```python
from build123d import *

# Parameters (mm, degrees)
SKETCH_1_R          = 6
EXTRUDE_1_DEPTH     = 3
FILLET_1_R          = 2
SKETCH_2_R          = 1.515
CUT_EXTRUDE_1_DEPTH = 10
CUT_EXTRUDE_2_DEPTH = 10
FILLET_2_R          = 1.2


with BuildPart() as part:
    # 草图1 → 凸台-拉伸1 (new body)
    with BuildSketch(Plane.XY):
        with BuildLine():
            Line((-20, -45), (20, -45))
            Line((20, -45), (20, -39))
            Line((20, -39), (12.287533689, 2.294889071))
            ThreePointArc((12.287533689, 2.294889071), (0, 12.5), (-12.287533689, 2.294889071))
            Line((-12.287533689, 2.294889071), (-20, -39))
            Line((-20, -39), (-20, -45))
        make_face()
        Circle(SKETCH_1_R, mode=Mode.SUBTRACT)
    extrude(amount=EXTRUDE_1_DEPTH)

    # 圆角1
    fillet_1_edges = [part.edges().sort_by_distance(p)[0] for p in [
        (20, -39, 1.5),
        (20, -45, 1.5),
        (-20, -45, 1.5),
        (-20, -39, 1.5),
    ]]
    fillet(fillet_1_edges, radius=FILLET_1_R)

    # 草图2 → 切除-拉伸1 (cut)
    with BuildSketch(Plane.XY.offset(3)):
        with Locations((-5, -42)):
            Circle(SKETCH_2_R)
        with Locations((15, -42)):
            Circle(SKETCH_2_R)
    extrude(amount=-CUT_EXTRUDE_1_DEPTH, mode=Mode.SUBTRACT)

    # 草图3 → 切除-拉伸2 (cut)
    with BuildSketch(Plane.XY.offset(3)):
        with BuildLine():
            Line((-8.849829987, -6.53303216), (-14.913543956, -39))
            Line((-14.913543956, -39), (14.913543956, -39))
            Line((14.913543956, -39), (8.849829987, -6.53303216))
            ThreePointArc((8.849829987, -6.53303216), (0, -11), (-8.849829987, -6.53303216))
        make_face()
    extrude(amount=-CUT_EXTRUDE_2_DEPTH, mode=Mode.SUBTRACT)

    # 圆角2
    fillet_2_edges = [part.edges().sort_by_distance(p)[0] for p in [
        (-8.849829987, -6.53303216, 1.5),
        (8.849829987, -6.53303216, 1.5),
        (14.913543956, -39, 1.5),
        (-14.913543956, -39, 1.5),
    ]]
    fillet(fillet_2_edges, radius=FILLET_2_R)


solid = part.part
```
Input: part model. Units: mm. Frame: model coordinates. A direction names the side the tool comes from. Round coordinates to 2 decimals unless told otherwise and drop trailing zeros. Write each loop counter-clockwise with the first axis right and the second up, starting at its lowest first coordinate (ties: lowest second). Pieces come first, ordered by that corner, then holes. Notation, with made-up numbers: M 50,39.5 L 73,39.5 A13 ccw 73,46.5 Z; hole C 71,-38 d7. An arc over 180 degrees is marked long. Write each question's results on one line, items separated by ' | '.
Q1. Access query for faces 1 (the face through (0, -11, 2)), 2 (the face through (20, -41, 1)). Directions: +Z, -Z, +X, -X, +Y, -Y. A direction counts if a zero-diameter tool reaches every point of the face in a straight line with its end or side. Return the directions, or none.
Results:
face 1: +Z, -Z | face 2: +Z, -Z, +X, +Y, -Y
Q2. Draft query along X for faces 3 (the face through (-19.4, -44.43, 1.52)), 4 (the face through (0, -39, 2)), 5 (the face through (0, -9, 0)). Return one class per face: released by +X, released by -X, zero draft, split by the parting line, or undercut.
Results:
face 3: released by -X | face 4: undercut | face 5: zero draft
Q3. Line query: line 1 along Y through (x, z) = (0, 1.7); line 2 along Y through (x, z) = (-5, 1.45) (3 decimals); line 3 along Y through (x, z) = (4, 2.1). Output: solid intervals per line, ascending.
Results:
line 1: y = -45 to -39, -11 to -6, 6 to 12.5 | line 2: y = -45 to -43.515, -40.485 to -39, -9.798 to -3.317, 3.317 to 11.456 | line 3: y = -45 to -39, -10.25 to -4.47, 4.47 to 11.84
Q4. Pin query (flat end, axial travel): P1, Ø6, axis at x = -12.5, y = -28.5, coming from the +Z side; P2, Ø1, axis at y = -16, z = 1, coming from the -X side; P3, Ø1.5, axis at x = -1.5, z = 1, coming from the +Y side; P4, Ø1.5, axis at y = -23.5, z = 0.5, coming from the +X side. Return the tip coordinate at first contact, or that it passes through.
Results:
P1: stops at z = 3 | P2: stops at x = -15.8 | P3: stops at y = 12.48 | P4: stops at x = 17.25
Q5. Section query B-B (x = 0). Return loops of the section in (y, z), and give its area (3 significant figures).
Results:
outline: M -45,0 L -39,0 L -39,3 L -45,3 Z; M -11,0 L -6,0 L -6,3 L -11,3 Z; M 6,0 L 12.5,0 L 12.5,3 L 6,3 Z | area: 52.5 mm^2
Q6. Section query C-C (z = 0.7). Return loops of the section in (x, y) (3 decimals), and give its area (3 significant figures).
Results:
outline: M -20,-43 A2 ccw -18,-45 L 18,-45 A2 ccw 20,-43 L 20,-39.185 A2 ccw 19.966,-38.818 L 12.288,2.295 A12.5 ccw -12.288,2.295 L -19.966,-38.818 A2 ccw -20,-39.185 Z; hole M -14.648,-37.58 A1.2 ccw -13.469,-39 L 13.469,-39 A1.2 ccw 14.648,-37.58 L 9.291,-8.893 A1.2 ccw 7.313,-8.217 A11 cw -7.313,-8.217 A1.2 ccw -9.291,-8.893 Z; hole C -5,-42 d3.03; hole C 0,0 d12; hole C 15,-42 d3.03 | area: 920 mm^2
Q7. Section query A-A (y = -42). Return loops of the section in (x, z) (3 decimals).
Results:
outline: M -20,0 L -6.515,0 L -6.515,3 L -20,3 Z; M -3.485,0 L 13.485,0 L 13.485,3 L -3.485,3 Z; M 16.515,0 L 20,0 L 20,3 L 16.515,3 Z
Q8. Section query D-D (x = 10). Return loops of the section in (y, z).
Results:
outline: M -45,0 L -39,0 L -39,3 L -45,3 Z; M -12.69,0 L 7.5,0 L 7.5,3 L -12.69,3 Z
